```python
from build123d import *

# Parameters (mm, degrees)
SKETCH_1_W          = 60
SKETCH_1_H          = 60
EXTRUDE_1_DEPTH     = 26.7
SKETCH_2_R          = 25
CUT_EXTRUDE_1_DEPTH = 3
SKETCH_3_R          = 7
CUT_EXTRUDE_2_DEPTH = 49.597222143
SKETCH_4_R          = 1.65
CUT_EXTRUDE_3_DEPTH = 10
SKETCH_5_R          = 30
EXTRUDE_2_DEPTH     = 36.3
SKETCH_6_W          = 60
SKETCH_6_H          = 60
EXTRUDE_3_DEPTH     = 8
SKETCH_7_R          = 25
EXTRUDE_4_DEPTH     = 7.2
SKETCH_8_R          = 8
EXTRUDE_5_DEPTH     = 22.5
SKETCH_9_R          = 2.5
CUT_EXTRUDE_4_DEPTH = 8
EXTRUDE_6_DEPTH     = 10
CHAMFER_1_SIZE      = 2
FILLET_1_R          = 1
SKETCH_11_R         = 8.5
EXTRUDE_7_DEPTH     = 1


with BuildPart() as part:
    # 草图1 → 凸台-拉伸1 (new body)
    with BuildSketch(Plane.XY):
        Rectangle(SKETCH_1_W, SKETCH_1_H)
    extrude(amount=EXTRUDE_1_DEPTH)

    # 草图2 → 切除-拉伸1 (cut)
    with BuildSketch(Plane(origin=(0, 0, 0), x_dir=(-1, 0, 0), z_dir=(0, 0, -1))):
        Circle(SKETCH_2_R)
    extrude(amount=-CUT_EXTRUDE_1_DEPTH, mode=Mode.SUBTRACT)

    # 草图3 → 切除-拉伸2 (cut, through all)
    with BuildSketch(Plane(origin=(0, 0, 3), x_dir=(-1, 0, 0), z_dir=(0, 0, -1))):
        Circle(SKETCH_3_R)
    extrude(amount=-CUT_EXTRUDE_2_DEPTH, mode=Mode.SUBTRACT)

    # 草图4 → 切除-拉伸3 (cut)
    with BuildSketch(Plane(origin=(0, 0, 0), x_dir=(-1, 0, 0), z_dir=(0, 0, -1))):
        with Locations((24.748737342, 24.748737342)):
            Circle(SKETCH_4_R)
        with Locations((-24.748737342, 24.748737342)):
            Circle(SKETCH_4_R)
        with Locations((24.748737342, -24.748737342)):
            Circle(SKETCH_4_R)
        with Locations((-24.748737342, -24.748737342)):
            Circle(SKETCH_4_R)
    extrude(amount=-CUT_EXTRUDE_3_DEPTH, mode=Mode.SUBTRACT)

    # 草图5 → 凸台-拉伸2 (add)
    with BuildSketch(Plane.XY.offset(26.7)):
        Circle(SKETCH_5_R)
    extrude(amount=EXTRUDE_2_DEPTH)

    # 草图6 → 凸台-拉伸3 (add)
    with BuildSketch(Plane.XY.offset(63)):
        Rectangle(SKETCH_6_W, SKETCH_6_H)
    extrude(amount=EXTRUDE_3_DEPTH)

    # 草图7 → 凸台-拉伸4 (add)
    with BuildSketch(Plane.XY.offset(71)):
        with Locations(Location((0, 0, 0), (0, 0, 180))):
            Circle(SKETCH_7_R)
    extrude(amount=EXTRUDE_4_DEPTH)

    # 草图8 → 凸台-拉伸5 (add)
    with BuildSketch(Plane.XY.offset(78.2)):
        with Locations(Location((0, 0, 0), (0, 0, 180))):
            Circle(SKETCH_8_R)
    extrude(amount=EXTRUDE_5_DEPTH)

    # 草图9 → 切除-拉伸4 (cut)
    with BuildSketch(Plane.XY.offset(71)):
        with Locations((-24.748737342, 24.748737342)):
            Circle(SKETCH_9_R)
        with Locations((24.748737342, 24.748737342)):
            Circle(SKETCH_9_R)
        with Locations((24.748737342, -24.748737342)):
            Circle(SKETCH_9_R)
        with Locations((-24.748737342, -24.748737342)):
            Circle(SKETCH_9_R)
    extrude(amount=-CUT_EXTRUDE_4_DEPTH, mode=Mode.SUBTRACT)

    # 草图10 → 凸台-拉伸6 (add)
    with BuildSketch(Plane(origin=(0, 0, 0), x_dir=(1, 0, 0), z_dir=(0, 1, 0))):
        with BuildLine():
            Line((2.5, -84.7), (2.5, -95.7))
            ThreePointArc((2.5, -95.7), (0, -98.2), (-2.5, -95.7))
            Line((-2.5, -95.7), (-2.5, -84.7))
            ThreePointArc((-2.5, -84.7), (0, -82.2), (2.5, -84.7))
        make_face()
    extrude(amount=EXTRUDE_6_DEPTH)

    # 倒角1
    chamfer_1_edges = [part.edges().sort_by_distance(p)[0] for p in [
        (-30, 30, 67),
        (-30, -30, 67),
        (30, -30, 67),
        (30, 30, 67),
        (30, -30, 13.35),
        (-30, -30, 13.35),
        (-30, 30, 13.35),
        (30, 30, 13.35),
    ]]
    chamfer(chamfer_1_edges, length=CHAMFER_1_SIZE)

    # 圆角1
    fillet_1_edges = [part.edges().sort_by_distance(p)[0] for p in [
        (8, 0, 100.7),
    ]]
    fillet(fillet_1_edges, radius=FILLET_1_R)

    # 草图11 → 凸台-拉伸7 (add)
    with BuildSketch(Plane.XY.offset(78.2)):
        Circle(SKETCH_11_R)
    extrude(amount=EXTRUDE_7_DEPTH)


solid = part.part
```
Source: CAD feature listing. Evaluate the final solid. Frame: model axes, mm. A direction names the side the tool comes from. Round coordinates to 2 decimals unless told otherwise and drop trailing zeros. Loops run counter-clockwise (first coordinate to the right, second up) from the corner with the lowest first, then second, coordinate; pieces in that order, holes last. Notation, with made-up numbers: M 87.25,28.5 L 123.25,28.5 A19 ccw 123.25,40.5 Z; hole C 71.5,32 d5. An arc over 180 degrees is marked long. Use a Markdown table: item, result. Add a question column.
1. Section query B-B on y = -13. Return the cut outline in (x, z), then the cut area to 3 significant figures.
2. Mould query, pull axis Z, two halves, no side actions, for faces 1 (the flat face through (23, -24, 26.7)), 2 (the flat face through (-27, 0, 0)), 3 (the flat face through (-24, 23, 26.7)), 4 (the flat face through (30, 0, 67)). Classes: pulls with the +Z half, pulls with the -Z half, needs draft (parallel to the pull), parting line crosses it, or undercut.
3. Section query C-C on x = 13.5. Return the cut outline in (y, z).
4. Section query A-A on z = 19.5. Return the cut outline in (x, y), then the cut area to 3 significant figures.
5. Contact query for flat-ended pins moving along their axis: P1, Ø0.7, axis at y = 9, z = 89.5, coming from the +X side; P2, Ø4, axis at x = 24.75, y = 24.75, coming from the +Z side; P3, Ø5.5, axis at x = 1, z = 86, coming from the +Y side. Output: stop coordinate, or through.
6. Reachability of faces 5 (the cylindrical face through (-6.466, -2.681, 14.684)), 6 (the cylindrical face through (-23.405, -22.641, 67.056)), 7 (the flat face through (-22.8, -22.7, 63)) from +Z, -Z, +X, -X, +Y, -Y: full face, straight path, thin tool, end or side. Return the list, or none.
7. Line query: line 1 (Z direction, x = -17.5, y = -24.5); line 2 (Z direction, x = -8.5, y = 8); line 3 (Z direction, x = -1, y = 1). Output: solid intervals per line, ascending.
8. Section query D-D on z = 37.5. Return the cut outline in (x, y), then the cut area to 3 significant figures.
Reported:
| question | item | result |
|---|---|---|
| 1 | outline | M -30,0 L -21.35,0 L -21.35,3 L 21.35,3 L 21.35,0 L 30,0 L 30,26.7 L 27.04,26.7 L 27.04,63 L 30,63 L 30,71 L 21.35,71 L 21.35,78.2 L -21.35,78.2 L -21.35,71 L -30,71 L -30,63 L -27.04,63 L -27.04,26.7 L -30,26.7 Z |
| 1 | area | 4,220 mm² |
| 2 | face 1 | undercut |
| 2 | face 2 | pulls with the -Z half |
| 2 | face 3 | undercut |
| 2 | face 4 | needs draft |
| 3 | outline | M -30,0 L -21.04,0 L -21.04,3 L 21.04,3 L 21.04,0 L 30,0 L 30,26.7 L 26.79,26.7 L 26.79,63 L 30,63 L 30,71 L 21.04,71 L 21.04,78.2 L -21.04,78.2 L -21.04,71 L -30,71 L -30,63 L -26.79,63 L -26.79,26.7 L -30,26.7 Z |
| 4 | outline | M -30,-28 L -28,-30 L 28,-30 L 30,-28 L 30,28 L 28,30 L -28,30 L -30,28 Z; hole C 0,0 d14 |
| 4 | area | 3,440 mm² |
| 5 | P1 | stops at x = 2.5 |
| 5 | P2 | stops at z = 26.7 |
| 5 | P3 | stops at y = 10 |
| 6 | face 5 | -Z |
| 6 | face 6 | +Z |
| 6 | face 7 | -X, -Y |
| 7 | line 1 | z = 0 to 26.7, 63 to 71 |
| 7 | line 2 | z = 3 to 78.2 |
| 7 | line 3 | z = 26.7 to 100.7 |
| 8 | outline | C 0,0 d60 |
| 8 | area | 2,830 mm² |
